CAD build for the part. Positions are in the model's coordinates, mm. A direction names the side the tool comes from. Round coordinates to 2 decimals unless told otherwise and drop trailing zeros. Order: outer loops, then holes, each group sorted by start corner. A loop starts at its lowest first (then second) coordinate and runs counter-clockwise, first axis right, second up. Notation, with made-up numbers: (49.25, 22.5) -> (107.25, 22.5) arc R22 cw to (107.25, 29.5) -> close; hole circle Ø3 at (26.5, -31). An arc over 180 degrees is marked (long way). Return JSON: item names as keys, results as strings. Group by question number.
Q1. Which spindle directions (+Z, -Z, +X, -X, +Y, -Y) get a long thin tool onto all of the face, cutting with end or side? Do faces 4 (the cylindrical face through (-0.9, 0.49, 2.86)), 5 (the cylindrical face through (19.233, 2.465, 0.26)). Say none if no direction does.
Q2. Cut at B-B (x = 0). Write the cut outline in (y, z).
Q3. Mould opens along X. For faces 1 (the cylindrical face through (0.9, 7.86, 2.86)), 2 (the flat face through (0, 10.8, 0)), 3 (the cylindrical face through (-15.267, 2.465, 0.26)) say: +X half, -X half, draft (parallel to the pull), parting line (faces both ways), or undercut.
Q4. Cut at A-A (z = 0). Write the cut outline in (x, y).
Q5. Flat gauge pins, fed straight in: pin 1 (6 mm diameter, centred on x = -5.5, y = 4, fed in from -Z); pin 2 (6.5 mm diameter, centred on x = -1, z = 0, fed in from -Y); pin 3 (4.5 mm diameter, centred on x = -17.25, z = 0, fed in from +Y); pin 4 (5 mm diameter, centred on x = 0, z = 0, fed in from -Y). Where does each tip first touch, or does it go through?
Q6. Cut at C-C (y = 3). Write the cut outline in (x, z) (3 decimals).
Q7. Probe line 1 along X through (y, z) = (0.7, 0); line 2 along X through (y, z) = (3, 0); line 3 along Y through (x, z) = (2.5, 24). List the from-to ranges inside material, lowest first.
Q8. Cut at D-D (x = 17.25). Write the cut outline in (y, z), then the cut area to 3 significant figures.
from build123d import *

# Parameters (mm, degrees)
SKETCH_1_R          = 29.5
EXTRUDE_1_DEPTH     = 5
SKETCH_2_R          = 3
EXTRUDE_2_DEPTH     = 5.8
SKETCH_3_R          = 2
CUT_EXTRUDE_1_DEPTH = 5
SKETCH_4_R          = 3
CUT_EXTRUDE_2_DEPTH = 1


with BuildPart() as part:
    # 草图1 → 凸台-拉伸1 (new body)
    with BuildSketch(Plane(origin=(0, 0, 0), x_dir=(1, 0, 0), z_dir=(0, 1, 0))):
        with Locations(Location((0, 0, 0), (0, 0, 270))):
            Circle(SKETCH_1_R)
    extrude(amount=EXTRUDE_1_DEPTH)

    # 草图2 → 凸台-拉伸2 (add)
    with BuildSketch(Plane(origin=(0, 5, 0), x_dir=(1, 0, 0), z_dir=(0, 1, 0))):
        with Locations(Location((0, 0, 0), (0, 0, 270))):
            Circle(SKETCH_2_R)
    extrude(amount=EXTRUDE_2_DEPTH)

    # 草图3 → 切除-拉伸1 (cut)
    with BuildSketch(Plane.XZ):
        with Locations(Location((17.25, 0, 0), (0, 0, 270))):
            Circle(SKETCH_3_R)
        with Locations(Location((8.625, -14.938938215, 0), (0, 0, 270))):
            Circle(SKETCH_3_R)
        with Locations(Location((-8.625, -14.938938215, 0), (0, 0, 270))):
            Circle(SKETCH_3_R)
        with Locations(Location((-17.25, 0, 0), (0, 0, 270))):
            Circle(SKETCH_3_R)
        with Locations(Location((-8.625, 14.938938215, 0), (0, 0, 270))):
            Circle(SKETCH_3_R)
        with Locations(Location((8.625, 14.938938215, 0), (0, 0, 270))):
            Circle(SKETCH_3_R)
    extrude(amount=-CUT_EXTRUDE_1_DEPTH, mode=Mode.SUBTRACT)

    # 草图4 → 切除-拉伸2 (cut)
    with BuildSketch(Plane.XZ):
        with Locations(Location((0, 0, 0), (0, 0, 90))):
            Circle(SKETCH_4_R)
    extrude(amount=-CUT_EXTRUDE_2_DEPTH, mode=Mode.SUBTRACT)


solid = part.part
Solution:
{
 "1": {"face 4": "-Y", "face 5": "+Y, -Y"},
 "2": {"outline": "(0, -29.5) -> (5, -29.5) -> (5, -3) -> (10.8, -3) -> (10.8, 3) -> (5, 3) -> (5, 29.5) -> (0, 29.5) -> (0, 3) -> (1, 3) -> (1, -3) -> (0, -3) -> close"},
 "3": {"face 1": "parting line", "face 2": "draft", "face 3": "undercut"},
 "4": {"outline": "(-29.5, 0) -> (-19.25, 0) -> (-19.25, 5) -> (-29.5, 5) -> close; (-15.25, 0) -> (-3, 0) -> (-3, 1) -> (3, 1) -> (3, 0) -> (15.25, 0) -> (15.25, 5) -> (3, 5) -> (3, 10.8) -> (-3, 10.8) -> (-3, 5) -> (-15.25, 5) -> close; (19.25, 0) -> (29.5, 0) -> (29.5, 5) -> (19.25, 5) -> close"},
 "5": {"pin 1": "stops at z = -29.39", "pin 2": "stops at y = 0", "pin 3": "stops at y = 5", "pin 4": "stops at y = 1"},
 "6": {"outline": "circle Ø59 at (0, 0); hole circle Ø4 at (-17.25, 0); hole circle Ø4 at (-8.625, -14.939); hole circle Ø4 at (-8.625, 14.939); hole circle Ø4 at (8.625, -14.939); hole circle Ø4 at (8.625, 14.939); hole circle Ø4 at (17.25, 0)"},
 "7": {"line 1": "x = -29.5 to -19.25, -15.25 to -3, 3 to 15.25, 19.25 to 29.5", "line 2": "x = -29.5 to -19.25, -15.25 to 15.25, 19.25 to 29.5", "line 3": "y = 0 to 5"},
 "8": {"outline": "(0, -23.93) -> (5, -23.93) -> (5, -2) -> (0, -2) -> close; (0, 2) -> (5, 2) -> (5, 23.93) -> (0, 23.93) -> close", "area": "219 mm²"}
}
